Study the drawing (mm; zero at the part's minimum x, y, z) and answer. Coordinates: 2 decimals unless noted, no trailing zeros. Order: outer loops, then holes, each group sorted by start corner. A loop starts at its lowest first (then second) coordinate and runs counter-clockwise, first axis right, second up. Notation, with made-up numbers: (84, 73.5) -> (88, 73.5) arc R4 ccw to (88, 78.5) -> close; hole circle Ø6 at (-22.5, -32). An arc over 180 degrees is marked (long way). One line per question, with ' | ' between items.
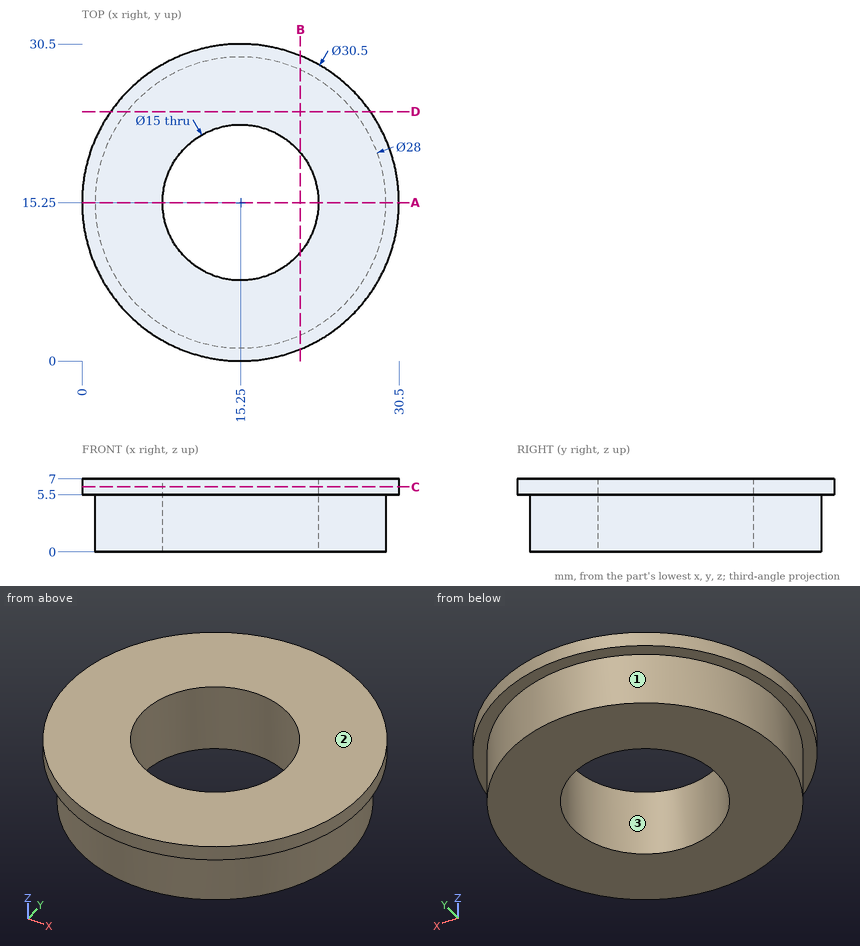
Item 1: Determine the mould class of the marked faces 1, 2 and 3 for opening direction X: pulls with the +X half, pulls with the -X half, needs draft (parallel to the pull), parting line crosses it, or undercut.
Computed values:
face 1: parting line crosses it | face 2: needs draft | face 3: undercut
Item 2: Section A-A, the plane y = 15.25 is taken. Give the vertices of the cut face in (x, z), plus the area to 4 significant figures.
Computed values:
outline: (0, 5.5) -> (1.25, 5.5) -> (1.25, 0) -> (7.75, 0) -> (7.75, 7) -> (0, 7) -> close; (22.75, 0) -> (29.25, 0) -> (29.25, 5.5) -> (30.5, 5.5) -> (30.5, 7) -> (22.75, 7) -> close | area: 94.75 mm^2
Item 3: Each of these flat-tipped pins is pushed along its axis until it touches: pin 1 Ø1 at (x, z) = (3, 0.5) entering from -Y; pin 2 Ø4 at (x, z) = (17, 4) entering from -Y; pin 3 Ø1.5 at (y, z) = (26.5, 5.5) entering from -X. Where does it stop, or does it pass through?
Computed values:
pin 1: stops at y = 7.64 | pin 2: stops at y = 0.01 | pin 3: stops at x = 4.19
Item 4: Section C-C, the plane z = 6.25 is taken. Give the vertices of the cut face in (x, y), plus the area to 3 significant figures.
Computed values:
outline: circle Ø30.5 at (15.25, 15.25); hole circle Ø15 at (15.25, 15.25) | area: 554 mm^2
Item 5: Section D-D, the plane y = 24 is taken. Give the vertices of the cut face in (x, z), plus the area to 3 significant figures.
Computed values:
outline: (2.76, 5.5) -> (4.32, 5.5) -> (4.32, 0) -> (26.18, 0) -> (26.18, 5.5) -> (27.74, 5.5) -> (27.74, 7) -> (2.76, 7) -> close | area: 158 mm^2
Item 6: Find the intervals of material crossed by L1, parallel to Y at x = 15.25, z = 2.5; L2, parallel to X at y = 9.5, z = 4.75; L3, parallel to Y at x = 10, z = 3.75, in increasing order.
Computed values:
L1: y = 1.25 to 7.75, 22.75 to 29.25 | L2: x = 2.49 to 10.43, 20.07 to 28.01 | L3: y = 2.27 to 9.89, 20.61 to 28.23
Item 7: Section B-B, the plane x = 21 is taken. Give the vertices of the cut face in (y, z), plus the area to 3 significant figures.
Computed values:
outline: (1.13, 5.5) -> (2.49, 5.5) -> (2.49, 0) -> (10.43, 0) -> (10.43, 7) -> (1.13, 7) -> close; (20.07, 0) -> (28.01, 0) -> (28.01, 5.5) -> (29.37, 5.5) -> (29.37, 7) -> (20.07, 7) -> close | area: 115 mm^2
